Read the model definition and answer for the solid it produces. Units are mm, in the model's axes. Face numbers are marked on the shaded views. A direction names the side the tool comes from. Coordinates: 2 decimals unless noted, no trailing zeros. Write each loop counter-clockwise with the first axis right and the second up, starting at its lowest first coordinate (ties: lowest second). Pieces come first, ordered by that corner, then holes. Notation, with made-up numbers: (77, -5) - (112, -5) arc R17 ccw to (112, 16) - close; hole circle Ø9 at (2, -4). An arc over 180 degrees is marked (long way). Use a Markdown table: item, result.
Autodesk Inventor part; units mm, degrees
ref_plane "YZ Plane" through (0, 0, 0) normal (1, 0, 0) x (0, 1, 0)
ref_plane "XZ Plane" through (0, 0, 0) normal (0, 1, 0) x (-1, 0, 0)
ref_plane "XY Plane" through (0, 0, 0) normal (0, 0, 1) x (1, 0, 0)
sketch "Sketch1" plane through (0, 0, 0) normal (0, 1, 0) x (-1, 0, 0)
  circle A0 centre (0, 0) radius 1.5
  dimension "d0" = 3
extrude "Extrusion1" add sketch "Sketch1" along normal blind 4.75
sketch "Sketch2" plane through (0, 4.75, 0) normal (0, 1, 0) x (1, 0, 0)
  circle A0 centre (0, 0) radius 2.5
  dimension "d3" = 5
extrude "Extrusion2" add sketch "Sketch2" along normal blind 2
fillet "Fillet1" radius 0.5 2 edges at (-2.5, 6.75, 0) (-2.5, 4.75, 0)
sketch "Sketch3" plane through (0, 6.75, 0) normal (0, 1, 0) x (1, 0, 0)
  line L0 (0.5, -1.5) -> (-0.5, -1.5)
  line L1 (-0.5, -1.5) -> (-0.5, 1.5)
  line L2 (-0.5, 1.5) -> (0.5, 1.5)
  line L3 (0.5, 1.5) -> (0.5, -1.5)
  line L4 (0.5, -1.5) -> (-0.5, 1.5) construction
  line L5 (-0.5, -1.5) -> (0.5, 1.5) construction
  line L6 (-1.5, -0.5) -> (1.5, -0.5)
  line L7 (1.5, -0.5) -> (1.5, 0.5)
  line L8 (1.5, 0.5) -> (-1.5, 0.5)
  line L9 (-1.5, 0.5) -> (-1.5, -0.5)
  line L10 (-1.5, -0.5) -> (1.5, 0.5) construction
  line L11 (1.5, -0.5) -> (-1.5, 0.5) construction
  point P0 (0, 0)
  point P1 (-0.5, -0.5)
  point P2 (0.5, -0.5)
  point P3 (0.5, 0.5)
  point P4 (-0.5, 0.5)
  dimension "d7" = 1
  dimension "d8" = 3
  dimension "d9" = 3
  dimension "d10" = 1
extrude "Extrusion3" cut sketch "Sketch3" against normal blind 1
thread "Thread1"
chamfer "Chamfer1" distance 0.25 angle 45 1 edges at (1.5, 0, 0)
properties part number "M3_Smaller_Bolt" material "Steel, Alloy"
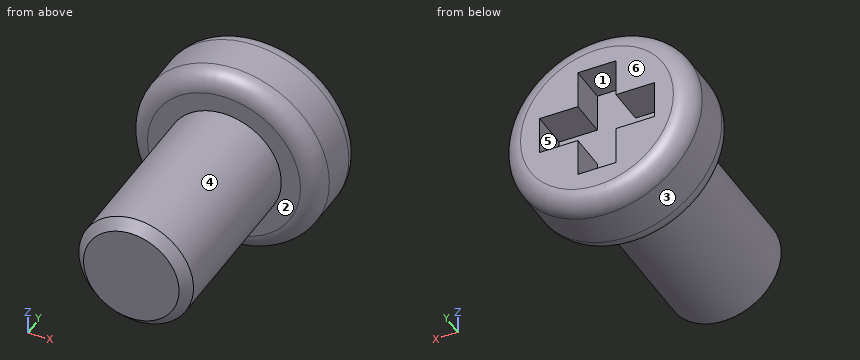
(1) A cutting plane is placed at A-A, the plane x = 0. Write down the section's boundary in (y, z).
Report:
| item | result |
|---|---|
| outline | (0, -1.25) - (0.25, -1.5) - (4.75, -1.5) - (4.75, -2) arc R0.5 ccw to (5.25, -2.5) - (6.25, -2.5) arc R0.5 ccw to (6.75, -2) - (6.75, -1.5) - (5.75, -1.5) - (5.75, 1.5) - (6.75, 1.5) - (6.75, 2) arc R0.5 ccw to (6.25, 2.5) - (5.25, 2.5) arc R0.5 ccw to (4.75, 2) - (4.75, 1.5) - (0.25, 1.5) - (0, 1.25) - close |
(2) For the marked faces 1, 2 and 3, determine the directions among +Z, -Z, +X, -X, +Y, -Y from which every point of the face is accessible in a straight line to the end or side of a thin tool.
Report:
| item | result |
|---|---|
| face 1 | +Y |
| face 2 | -Y |
| face 3 | +Y, -Y |
(3) The mould has two halves that part along X. Classify the marked faces 4, 5 and 6: pulls with the +X half, pulls with the -X half, needs draft (parallel to the pull), parting line crosses it, or undercut.
Report:
| item | result |
|---|---|
| face 4 | parting line crosses it |
| face 5 | undercut |
| face 6 | needs draft |
(4) A cutting plane is placed at B-B, the plane z = 0. Write down the section's boundary in (x, y), and give its area (3 significant figures).
Report:
| item | result |
|---|---|
| outline | (-2.5, 5.25) arc R0.5 ccw to (-2, 4.75) - (-1.5, 4.75) - (-1.5, 0.25) - (-1.25, 0) - (1.25, 0) - (1.5, 0.25) - (1.5, 4.75) - (2, 4.75) arc R0.5 ccw to (2.5, 5.25) - (2.5, 6.25) arc R0.5 ccw to (2, 6.75) - (1.5, 6.75) - (1.5, 5.75) - (-1.5, 5.75) - (-1.5, 6.75) - (-2, 6.75) arc R0.5 ccw to (-2.5, 6.25) - close |
| area | 21.0 mm² |
(5) Each of these flat-tipped pins is pushed along its axis until it touches: P1, Ø0.8, axis at y = 6, z = 1, coming from the +X side; P2, Ø1.1, axis at x = 1, y = 6.5, coming from the +Z side; P3, Ø0.5, axis at y = 6, z = 1, coming from the -X side. Where does it stop, or does it pass through?
Report:
| item | result |
|---|---|
| P1 | stops at x = 2.43 |
| P2 | stops at z = 2.45 |
| P3 | stops at x = -2.38 |
(6) A cutting plane is placed at C-C, the plane y = 2.5. Write down the section's boundary in (x, z), and give its area (3 significant figures).
Report:
| item | result |
|---|---|
| outline | circle Ø3 at (0, 0) |
| area | 7.07 mm² |
(7) Straight lines are drawn through the part: L1, parallel to X at y = 6, z = 0.1; L2, parallel to Z at x = -0.05, y = 1.25; L3, parallel to Z at x = 1, y = 6. For each, find the intervals that lie inside material, in ascending order.
Report:
| item | result |
|---|---|
| L1 | x = -2.5 to -1.5, 1.5 to 2.5 |
| L2 | z = -1.5 to 1.5 |
| L3 | z = -2.29 to -0.5, 0.5 to 2.29 |
